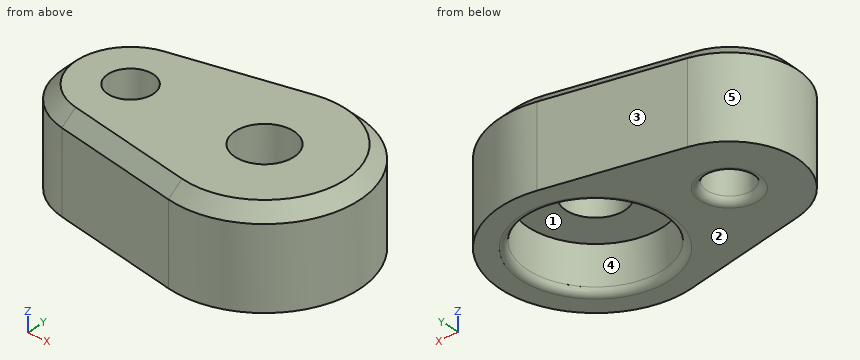
```python
from build123d import *

# Parameters (mm, degrees)
SKETCH1_R           = 2.175
SKETCH1_R_2         = 1.675
BOSS_EXTRUDE1_DEPTH = 7
SKETCH2_R           = 5
CUT_EXTRUDE1_DEPTH  = 3.4
CHAMFER1_SIZE       = 1
FILLET1_R           = 0.5


with BuildPart() as part:
    # Sketch1 → Boss-Extrude1 (new body)
    with BuildSketch(Plane.XY):
        with BuildLine():
            Line((-1.4, 6.85857128), (-11, 4.898979486))
            ThreePointArc((-11, 4.898979486), (-15, 0), (-11, -4.898979486))
            Line((-11, -4.898979486), (-1.4, -6.85857128))
            ThreePointArc((-1.4, -6.85857128), (7, 0), (-1.4, 6.85857128))
        make_face()
        Circle(SKETCH1_R, mode=Mode.SUBTRACT)
        with Locations((-10, 0)):
            Circle(SKETCH1_R_2, mode=Mode.SUBTRACT)
    extrude(amount=BOSS_EXTRUDE1_DEPTH)

    # Sketch2 → Cut-Extrude1 (cut)
    with BuildSketch(Plane(origin=(0, 0, 0), x_dir=(-1, 0, 0), z_dir=(0, 0, -1))):
        Circle(SKETCH2_R)
    extrude(amount=-CUT_EXTRUDE1_DEPTH, mode=Mode.SUBTRACT)

    # Chamfer1
    chamfer1_edges = [part.edges().sort_by_distance(p)[0] for p in [
        (-15, 0, 7),
        (-6.2, -5.878775383, 7),
        (7, 0, 7),
        (-6.2, 5.878775383, 7),
    ]]
    chamfer(chamfer1_edges, length=CHAMFER1_SIZE)

    # Fillet1
    fillet1_edges = [part.edges().sort_by_distance(p)[0] for p in [
        (-11.675, 0, 0),
        (5, 0, 0),
    ]]
    fillet(fillet1_edges, radius=FILLET1_R)


solid = part.part
```
Input: part model. Units: mm. Frame: model coordinates. Face numbers are marked on the shaded views. A direction names the side the tool comes from. Coordinates: 2 decimals unless noted, no trailing zeros. Order: outer loops, then holes, each group sorted by start corner. A loop starts at its lowest first (then second) coordinate and runs counter-clockwise, first axis right, second up. Notation, with made-up numbers: (80.25, -22) - (103.25, -22) arc R26 ccw to (103.25, 10) - close; hole circle Ø3 at (22.5, 20.5). An arc over 180 degrees is marked (long way). Return JSON: item names as keys, results as strings.
Q1. Cut plane A-A (x = 0). Return loops of the section in (y, z) (3 decimals), then the cut area to 3 significant figures.
The answers:
{"outline": "(-7, 0) - (-5.5, 0) arc R0.5 ccw to (-5, 0.5) - (-5, 3.4) - (-2.175, 3.4) - (-2.175, 7) - (-6, 7) - (-7, 6) - close; (2.175, 3.4) - (5, 3.4) - (5, 0.5) arc R0.5 ccw to (5.5, 0) - (7, 0) - (7, 6) - (6, 7) - (2.175, 7) - close", "area": "47.2 mm2"}
Q2. Access query for the marked faces 4 and 5. Directions: +Z, -Z, +X, -X, +Y, -Y. A direction counts if a zero-diameter tool reaches every point of the face in a straight line with its end or side. Return the directions, or none.
The answers:
{"face 4": "-Z", "face 5": "+Z, -Z, -X"}
Q3. Cut plane D-D (x = -10). Return loops of the section in (y, z) (3 decimals), then the cut area to 3 significant figures.
The answers:
{"outline": "(-5.103, 0) - (-2.175, 0) arc R0.5 ccw to (-1.675, 0.5) - (-1.675, 7) - (-4.082, 7) - (-5.103, 6) - close; (1.675, 0.5) arc R0.5 ccw to (2.175, 0) - (5.103, 0) - (5.103, 6) - (4.082, 7) - (1.675, 7) - close", "area": "46.9 mm2"}
Q4. Cut plane B-B (y = 0). Return loops of the section in (x, z) (3 decimals), then the cut area to 3 significant figures.
The answers:
{"outline": "(-15, 0) - (-12.175, 0) arc R0.5 ccw to (-11.675, 0.5) - (-11.675, 7) - (-14, 7) - (-15, 6) - close; (-8.325, 0.5) arc R0.5 ccw to (-7.825, 0) - (-5.5, 0) arc R0.5 ccw to (-5, 0.5) - (-5, 3.4) - (-2.175, 3.4) - (-2.175, 7) - (-8.325, 7) - close; (2.175, 3.4) - (5, 3.4) - (5, 0.5) arc R0.5 ccw to (5.5, 0) - (7, 0) - (7, 6) - (6, 7) - (2.175, 7) - close", "area": "79.7 mm2"}
Q5. Ray query, probe 1 along X at (y, z) = (-0.25, 5); probe 2 along Y at (x, z) = (0, 2.85); probe 3 along X at (y, z) = (1.5, 3.5) (3 decimals). Return the intervals inside material, ascending.
The answers:
{"probe 1": "x = -14.99 to -11.66, -8.34 to -2.16, 2.16 to 7", "probe 2": "y = -7 to -5, 5 to 7", "probe 3": "x = -14.77 to -10.745, -9.255 to -1.575, 1.575 to 6.837"}
Q6. Cut plane C-C (z = 2.5). Return loops of the section in (x, y) (3 decimals), then the cut area to 3 significant figures.
The answers:
{"outline": "(-11, -4.899) - (-1.4, -6.859) arc R7 ccw (long way) to (-1.4, 6.859) - (-11, 4.899) arc R5 ccw to start; hole circle Ø3.35 at (-10, 0); hole circle Ø10 at (0, 0)", "area": "151 mm2"}
Q7. First-contact query: pin 1 (2 mm diameter, centred on x = -7, z = 2, fed in from -Y); pin 2 (1.5 mm diameter, centred on x = -7, z = 2.5, fed in from +Y); pin 3 (8 mm diameter, centred on x = 0, y = 0, fed in from -Z). Flat tips, straight axial feed; report the tip coordinate or a pass-through.
The answers:
{"pin 1": "stops at y = -5.92", "pin 2": "stops at y = 5.87", "pin 3": "stops at z = 3.4"}
Q8. Draft query along X for the marked faces 1, 2 and 3. Return one class per face: +X half, -X half, draft (parallel to the pull), parting line (faces both ways), or undercut.
The answers:
{"face 1": "undercut", "face 2": "draft", "face 3": "-X half"}
